CAD build for the part. Positions are in the model's coordinates, mm. A direction names the side the tool comes from. Round coordinates to 2 decimals unless told otherwise and drop trailing zeros. Order: outer loops, then holes, each group sorted by start corner. A loop starts at its lowest first (then second) coordinate and runs counter-clockwise, first axis right, second up. Notation, with made-up numbers: (89.5, 71) - (134.5, 71) arc R25 ccw to (134.5, 109) - close; hole circle Ø7 at (50.5, -20.75). An arc over 180 degrees is marked (long way). Use one line per item in the form item = value. Start each with the question number.
from build123d import *

# Parameters (mm, degrees)
BASE_FLANGE1_DEPTH     = 1.5
SKETCHED_START         = -35
SKETCHED_BEND1_DEPTH   = 70
SKETCHED_BEND1_2_DEPTH = 70
CHAMFER1_SIZE          = 5
SKETCH7_R              = 2.5
CUT_EXTRUDE1_DEPTH     = 74.21454467


# Read off the part's stored shape, not the designer's step: Sketched Bend1
# Sheet-metal steps are written as plain solids
with BuildPart() as part:
    # Sketch1 → Base-Flange1 (new body)
    with BuildSketch(Plane(origin=(0, 0, 0), x_dir=(0, 1, 0), z_dir=(0, 0, 1))):
        Polygon((-30, -35), (30, -35), (52.5, -35), (52.5, 35), (30, 35), (-30, 35), (-52.5, 35), (-52.5, -35), align=None)
    extrude(amount=-BASE_FLANGE1_DEPTH)

    # Sketched Bend1 outline → Sketched Bend1 (cut)
    with BuildSketch(Plane.YZ.offset(SKETCHED_START)):
        with BuildLine():
            ThreePointArc((29.875223856, 0), (29.058564082, -1.086838938), (27.7634, -1.5))
            Line((27.7634, -1.5), (52.5, -1.5))
            Line((52.5, -1.5), (52.5, 0))
            Line((52.5, 0), (29.875223856, 0))
        make_face()
        with BuildLine():
            Line((-52.5, -1.5), (-27.7634, -1.5))
            ThreePointArc((-27.7634, -1.5), (-29.058564082, -1.086838938), (-29.875223856, 0))
            Line((-29.875223856, 0), (-52.5, 0))
            Line((-52.5, 0), (-52.5, -1.5))
        make_face()
    extrude(amount=SKETCHED_BEND1_DEPTH, mode=Mode.SUBTRACT)

    # Sketched Bend1 2 outline → Sketched Bend1 2 (add)
    with BuildSketch(Plane.YZ.offset(SKETCHED_START)):
        with BuildLine():
            Line((27.7634, 0), (29.875223856, 0))
            ThreePointArc((29.875223856, 0), (29.968585343, 0.363053267), (30, 0.7366))
            Line((30, 0.7366), (30, 23.138054181))
            Line((30, 23.138054181), (28.5, 23.138054181))
            Line((28.5, 23.138054181), (28.5, 0.7366))
            ThreePointArc((28.5, 0.7366), (28.284254855, 0.215745145), (27.7634, 0))
        make_face()
        with BuildLine():
            ThreePointArc((-30, 0.7366), (-29.968585343, 0.363053267), (-29.875223856, 0))
            Line((-29.875223856, 0), (-27.7634, 0))
            ThreePointArc((-27.7634, 0), (-28.284254855, 0.215745145), (-28.5, 0.7366))
            Line((-28.5, 0.7366), (-28.5, 23.138054181))
            Line((-28.5, 23.138054181), (-30, 23.138054181))
            Line((-30, 23.138054181), (-30, 0.7366))
        make_face()
    extrude(amount=SKETCHED_BEND1_2_DEPTH)

    # Chamfer1
    chamfer1_edges = [part.edges().sort_by_distance(p)[0] for p in [
        (35, -29.25, 23.138054181),
        (-35, -29.25, 23.138054181),
        (-35, 29.25, 23.138054181),
        (35, 29.25, 23.138054181),
    ]]
    chamfer(chamfer1_edges, length=CHAMFER1_SIZE)

    # Sketch7 → Cut-Extrude1 (cut, through all)
    with BuildSketch(Plane(origin=(0, 30, 0), x_dir=(-1, 0, 0), z_dir=(0, 1, 0))):
        with Locations(Location((-20, 12.5, 0), (0, 0, 90))):
            Circle(SKETCH7_R)
        with Locations(Location((20, 12.5, 0), (0, 0, 90))):
            Circle(SKETCH7_R)
    extrude(amount=-CUT_EXTRUDE1_DEPTH, mode=Mode.SUBTRACT)


solid = part.part
(1) Slice it at B-B (z = 12.5). Give the cut face in (x, y), and give its area (3 significant figures).
(2) Slice it at C-C (z = 2.25). Give the cut face in (x, y).
(3) Which spindle directions (+Z, -Z, +X, -X, +Y, -Y) get a long thin tool onto all of the face, cutting with end or side? Do faces 4 (the flat face through (0, -28.5, 12)), 5 (the flat face through (-32.47, -29.24, 20.67)). Say none if no direction does.
(4) Wall check: line 1 (X direction, y = -28.9, z = 12.5); line 2 (Y direction, x = 16.5, z = 8); line 3 (Z direction, x = -18, y = 2). Give the ranges that are in metal, low to high. Write a range as [from, to].
(5) Mould opens along X. For faces 1 (the flat face through (0, 29, 23.138)), 2 (the flat face through (32.465, -29.24, 20.673)), 3 (the cylindrical face through (-18, 29, 11)) say: pulls with the +X half, pulls with the -X half, needs draft (parallel to the pull), parting line crosses it, or undercut.
(6) Slice it at D-D (x = 28). Give the cut face in (y, z), and give its area (4 significant figures).
(7) Slice it at A-A (x = -20). Give the cut face in (y, z).
(8) Flat gauge pins, fed straight in: P1, Ø4, axis at x = -20, z = 12.5, coming from the +Y side; P2, Ø12, axis at x = 22, y = -16.5, coming from the +Z side. Where does each tip first touch, or does it go through?
Results list:
q1.outline = (-35, -30) - (-22.5, -30) - (-22.5, -28.5) - (-35, -28.5) - close; (-35, 28.5) - (-22.5, 28.5) - (-22.5, 30) - (-35, 30) - close; (-17.5, -30) - (17.5, -30) - (17.5, -28.5) - (-17.5, -28.5) - close; (-17.5, 28.5) - (17.5, 28.5) - (17.5, 30) - (-17.5, 30) - close; (22.5, -30) - (35, -30) - (35, -28.5) - (22.5, -28.5) - close; (22.5, 28.5) - (35, 28.5) - (35, 30) - (22.5, 30) - close
q1.area = 180 mm²
q2.outline = (-35, -30) - (35, -30) - (35, -28.5) - (-35, -28.5) - close; (-35, 28.5) - (35, 28.5) - (35, 30) - (-35, 30) - close
q3.face_4 = +Z, +X, -X
q3.face_5 = +Z, -X, +Y, -Y
q4.line_1 = [-35, -22.5], [-17.5, 17.5], [22.5, 35]
q4.line_2 = [-30, -28.5], [28.5, 30]
q4.line_3 = [-1.5, 0]
q5.face_1 = needs draft
q5.face_2 = pulls with the +X half
q5.face_3 = undercut
q6.outline = (-30, 0.74) arc R2.24 ccw to (-27.76, -1.5) - (27.76, -1.5) arc R2.24 ccw to (30, 0.74) - (30, 23.14) - (28.5, 23.14) - (28.5, 0.74) arc R0.74 cw to (27.76, 0) - (-27.76, 0) arc R0.74 cw to (-28.5, 0.74) - (-28.5, 23.14) - (-30, 23.14) - close
q6.area = 157.5 mm²
q7.outline = (-30, 0.74) arc R2.24 ccw to (-27.76, -1.5) - (27.76, -1.5) arc R2.24 ccw to (30, 0.74) - (30, 10) - (28.5, 10) - (28.5, 0.74) arc R0.74 cw to (27.76, 0) - (-27.76, 0) arc R0.74 cw to (-28.5, 0.74) - (-28.5, 10) - (-30, 10) - close; (-30, 15) - (-28.5, 15) - (-28.5, 23.14) - (-30, 23.14) - close; (28.5, 15) - (30, 15) - (30, 23.14) - (28.5, 23.14) - close
q8.P1 = through
q8.P2 = 0
